Autodesk Inventor part; units mm, degrees
ref_plane "YZ Plane" through (0, 0, 0) normal (1, 0, 0) x (0, 1, 0)
ref_plane "XZ Plane" through (0, 0, 0) normal (0, 1, 0) x (-1, 0, 0)
ref_plane "XY Plane" through (0, 0, 0) normal (0, 0, 1) x (1, 0, 0)
sketch "草圖1" plane through (0, 0, 0) normal (0, 0, 1) x (1, 0, 0)
  circle A0 centre (0, 0) radius 93.5
  dimension "d0" = 187
extrude "擠出1" add sketch "草圖1" along normal blind 12
hole "孔1" at (0, 0, 12) direction (0, 0, -1) diameter 50 end through all counterbore diameter 50.8 counterbore depth 10
sketch "草圖2" plane through (0, 0, 12) normal (0, 0, 1) x (1, 0, 0)
  circle A0 centre (0, 0) radius 80 construction
  line L0 (0, 0) -> (56.5685, 56.5685) construction
  line L1 (0, 0) -> (80, 0) construction
  point P0 (0, 80)
  point P1 (-80, 0)
  point P2 (0, -80)
  point P3 (-56.5685, 56.5685)
  point P4 (-56.5685, -56.5685)
  point P5 (56.5685, -56.5685)
  dimension "d12" = 160
  dimension "d13" = 45
hole "孔2" at (0, 80, 12) at (-80, 0, 12) at (80, 0, 12) at (0, -80, 12) at (56.5685, 56.5685, 12) at (-56.5685, 56.5685, 12) at (-56.5685, -56.5685, 12) at (56.5685, -56.5685, 12) direction (0, 0, -1) diameter 12 end through all
chamfer "倒角1" distance 1 angle 45 2 edges at (-93.5, 0, 12) (-93.5, 0, 0)
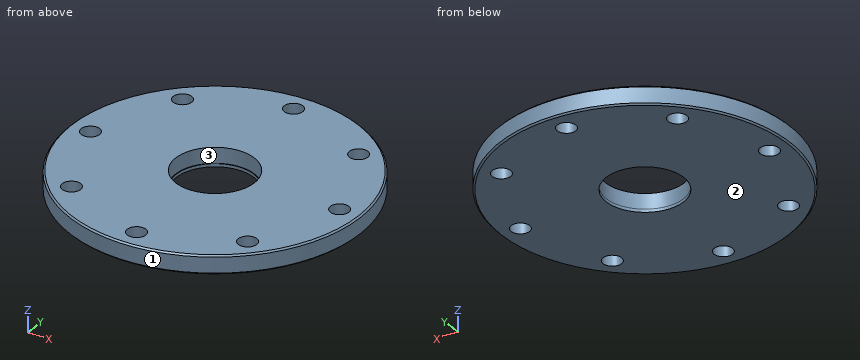
Could you check a few things on this model? Use its own coordinates, in mm. Face numbers are marked on the shaded views. Coordinates: 2 decimals unless noted, no trailing zeros. Write each loop counter-clockwise with the first axis right and the second up, starting at its lowest first coordinate (ties: lowest second). Pieces come first, ordered by that corner, then holes. Notation, with made-up numbers: (24, -4.5) - (53, -4.5) arc R30 ccw to (53, 26.5) - close; hole circle Ø8 at (-24.75, 74.25). An arc over 180 degrees is marked (long way). Put each result on its own line as item: value. Start each with the question number.
Q1. Please list where these lines run through material, in increasing order: L1, parallel to Y at x = 0, z = 7.75; L2, parallel to Y at x = -3, z = 5.75; L3, parallel to X at y = -51.5, z = 2.5.
Q2. Thinking about a two-plate mould opening in Y: for the marked faces 1, 2 and 3, which applies, pulls with the +Y half, pulls with the -Y half, needs draft (parallel to the pull), parting line crosses it, or undercut?
Q3. I want a section at A-A on x = 0. Write out the boundary of the cut face in (y, z), plus the area to 3 significant figures.
Q4. I'm going to push flat-ended pins straight in: P1, Ø5, axis at x = -42, z = 7, coming from the +Y side; P2, Ø7, axis at x = 0, y = 80, coming from the -Z side; P3, Ø1.5, axis at x = -24, z = 7.5, coming from the -Y side; P4, Ø4, axis at x = 11, z = 7.5, coming from the -Y side. Where does each tip first touch, or does it pass through?
Q5. I want a section at B-B on z = 8.5. Count the separate pieces of the cut face and the enclosed holes in it, plus the area to 3 significant figures.
Checks:
1. L1: -93.5 to -86, -74 to -25.4, 25.4 to 74, 86 to 93.5
1. L2: -93.45 to -85.2, -74.8 to -25.22, 25.22 to 74.8, 85.2 to 93.45
1. L3: -78.04 to -59.78, -53.36 to 53.36, 59.78 to 78.04
2. face 1: parting line crosses it
2. face 2: needs draft
2. face 3: undercut
3. outline: (-93.5, 1) - (-92.5, 0) - (-86, 0) - (-86, 12) - (-92.5, 12) - (-93.5, 11) - close; (-74, 0) - (-25, 0) - (-25, 2) - (-25.4, 2) - (-25.4, 12) - (-74, 12) - close; (25, 0) - (74, 0) - (74, 12) - (25.4, 12) - (25.4, 2) - (25, 2) - close; (86, 0) - (92.5, 0) - (93.5, 1) - (93.5, 11) - (92.5, 12) - (86, 12) - close
3. area: 1,350 mm²
4. P1: y = 84.75
4. P2: through
4. P3: y = -90.56
4. P4: y = -93.07
5. separate pieces: 1
5. enclosed holes: 9
5. area: 24,500 mm²
